For this review, take the finished solid that the model builds, in its own axes (mm). Round coordinates to 2 decimals unless told otherwise and drop trailing zeros. Loops run counter-clockwise (first coordinate to the right, second up) from the corner with the lowest first, then second, coordinate; pieces in that order, holes last.
1. Draft analysis for pull direction Z (two halves, no side actions). For faces 1 (the flat face through (7, 25, -1)), 2 (the flat face through (7, 0, 95)), 3 (the cylindrical face through (-440.46, -0.35, 3)), 4 (the flat face through (7, 0, -95)), state which applies: released by +Z, released by -Z, zero draft, split by the parting line, or undercut.
2. To check wall thickness, follow line 1 along Z through (x, y) = (-450, 4); line 2 along X through (y, z) = (5, -5). State the ranges of each line that lie inside material, in increasing order.
3. Consider section B-B on z = 0. State the section outline as (x, y) points, then the cut area to 3 significant figures.
4. Consider section A-A on x = -450. State the section outline as (y, z) points, then the cut area to 3 significant figures.
from build123d import *

# Parameters (mm, degrees)
F0_W     = 50
F0_H     = 190
F1_DEPTH = 500
F3_R     = 10
F4_DEPTH = 50.001


with BuildPart() as f1:
    # F0 (on Right) → F1 (new body, symmetric)
    with BuildSketch(Plane.YZ):
        Rectangle(F0_W, F0_H)
    extrude(amount=F1_DEPTH, both=True)

    # F3 (on face) → F4 (cut, through all)
    with BuildSketch(Plane.XZ.offset(25)):
        with Locations((-450, 0)):
            Circle(F3_R)
    extrude(amount=-F4_DEPTH, mode=Mode.SUBTRACT)


solid = f1.part
Resolved:
1. face 1: zero draft
1. face 2: released by +Z
1. face 3: undercut
1. face 4: released by -Z
2. line 1: z = -95 to -10, 10 to 95
2. line 2: x = -500 to -458.66, -441.34 to 500
3. outline: (-500, -25) - (-460, -25) - (-460, 25) - (-500, 25) - close; (-440, -25) - (500, -25) - (500, 25) - (-440, 25) - close
3. area: 49,000 mm2
4. outline: (-25, -95) - (25, -95) - (25, -10) - (-25, -10) - close; (-25, 10) - (25, 10) - (25, 95) - (-25, 95) - close
4. area: 8,500 mm2
